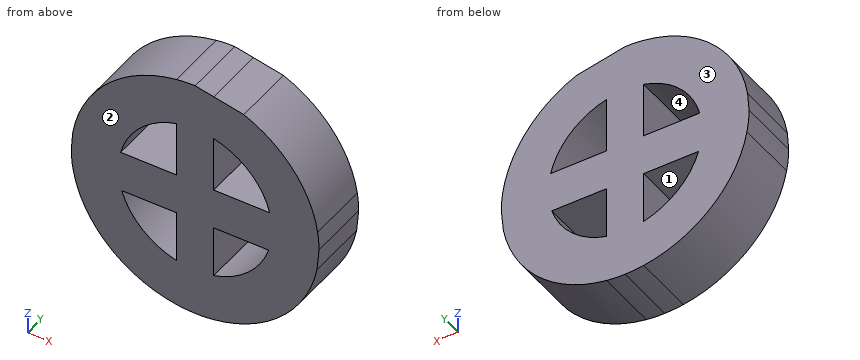
```python
from build123d import *

# Parameters (mm, degrees)
F1_DEPTH = 25


with BuildPart() as f1:
    # F0 (on Front) → F1 (new body)
    with BuildSketch(Plane.XZ):
        with BuildLine():
            Line((-7.5, 30.0790624854), (-7.5, 49.4342998332))
            ThreePointArc((-7.5, 49.4342998332), (-35.3553390593, 35.3553390593), (-49.4342998332, 7.5))
            Line((-49.4342998332, 7.5), (-30.0790624854, 7.5))
            ThreePointArc((-30.0790624854, 7.5), (-21.9203102168, 21.9203102168), (-7.5, 30.0790624854))
        make_face()
        with BuildLine():
            ThreePointArc((49.4342998332, 7.5), (39.5276683909, 30.6196576007), (19.6180084329, 45.9905832223))
            Line((19.6180084329, 45.9905832223), (7.5, 48.4671927359))
            Line((7.5, 48.4671927359), (7.5, 30.0790624854))
            ThreePointArc((7.5, 30.0790624854), (21.9203102168, 21.9203102168), (30.0790624854, 7.5))
            Line((30.0790624854, 7.5), (49.4342998332, 7.5))
        make_face()
        with BuildLine():
            ThreePointArc((7.5, -49.4342998332), (34.773891693, -35.9273775348), (49.1633315746, -9.1086128737))
            Line((49.1633315746, -9.1086128737), (29.631624517, -9.1086128737))
            ThreePointArc((29.631624517, -9.1086128737), (21.322038459, -22.502681528), (7.5, -30.0790624854))
            Line((7.5, -30.0790624854), (7.5, -49.4342998332))
        make_face()
        with BuildLine():
            Line((49.1633315746, -9.1086128737), (50, 0))
            Line((50, 0), (31, 0))
            ThreePointArc((31, 0), (30.6559974559, -4.6054120322), (29.631624517, -9.1086128737))
            Line((29.631624517, -9.1086128737), (49.1633315746, -9.1086128737))
        make_face()
        with BuildLine():
            ThreePointArc((50, 0), (49.8583743801, 3.7606520937), (49.4342998332, 7.5))
            Line((49.4342998332, 7.5), (30.0790624854, 7.5))
            ThreePointArc((30.0790624854, 7.5), (30.7689042464, 3.7781650939), (31, 0))
            Line((31, 0), (50, 0))
        make_face()
        with BuildLine():
            Line((7.5, 48.4671927359), (0, 50))
            Line((0, 50), (0, 31))
            ThreePointArc((0, 31), (3.7781650939, 30.7689042464), (7.5, 30.0790624854))
            Line((7.5, 30.0790624854), (7.5, 48.4671927359))
        make_face()
        with BuildLine():
            Line((-30.0790624854, 7.5), (-49.4342998332, 7.5))
            Line((-49.4342998332, 7.5), (-50, 0))
            Line((-50, 0), (-31, 0))
            ThreePointArc((-31, 0), (-30.7689042464, 3.7781650939), (-30.0790624854, 7.5))
        make_face()
        with BuildLine():
            Line((-31, 0), (-50, 0))
            ThreePointArc((-50, 0), (-49.790393545, -4.5734790515), (-49.1633315746, -9.1086128737))
            Line((-49.1633315746, -9.1086128737), (-29.631624517, -9.1086128737))
            ThreePointArc((-29.631624517, -9.1086128737), (-30.6559974559, -4.6054120322), (-31, 0))
        make_face()
        with BuildLine():
            Line((-29.631624517, -9.1086128737), (-49.1633315746, -9.1086128737))
            ThreePointArc((-49.1633315746, -9.1086128737), (-34.773891693, -35.9273775348), (-7.5, -49.4342998332))
            Line((-7.5, -49.4342998332), (-7.5, -30.0790624854))
            ThreePointArc((-7.5, -30.0790624854), (-21.322038459, -22.502681528), (-29.631624517, -9.1086128737))
        make_face()
        with BuildLine():
            Line((-7.5, -30.0790624854), (-7.5, -49.4342998332))
            ThreePointArc((-7.5, -49.4342998332), (-3.7606520937, -49.8583743801), (0, -50))
            Line((0, -50), (0, -31))
            ThreePointArc((0, -31), (-3.7781650939, -30.7689042464), (-7.5, -30.0790624854))
        make_face()
        with BuildLine():
            ThreePointArc((0, -50), (3.7606520937, -49.8583743801), (7.5, -49.4342998332))
            Line((7.5, -49.4342998332), (7.5, -30.0790624854))
            ThreePointArc((7.5, -30.0790624854), (3.7781650939, -30.7689042464), (0, -31))
            Line((0, -31), (0, -50))
        make_face()
        with BuildLine():
            Line((0, 31), (0, 50))
            ThreePointArc((0, 50), (-3.7606520937, 49.8583743801), (-7.5, 49.4342998332))
            Line((-7.5, 49.4342998332), (-7.5, 30.0790624854))
            ThreePointArc((-7.5, 30.0790624854), (-3.7781650939, 30.7689042464), (0, 31))
        make_face()
        with BuildLine():
            Line((-7.5, 7.5), (-30.0790624854, 7.5))
            ThreePointArc((-30.0790624854, 7.5), (-30.7689042464, 3.7781650939), (-31, 0))
            Line((-31, 0), (-7.5, 0))
            Line((-7.5, 0), (-7.5, 7.5))
        make_face()
        with BuildLine():
            Line((-7.5, -9.1086128737), (-7.5, 0))
            Line((-7.5, 0), (-31, 0))
            ThreePointArc((-31, 0), (-30.6559974559, -4.6054120322), (-29.631624517, -9.1086128737))
            Line((-29.631624517, -9.1086128737), (-7.5, -9.1086128737))
        make_face()
        with BuildLine():
            ThreePointArc((31, 0), (30.7689042464, 3.7781650939), (30.0790624854, 7.5))
            Line((30.0790624854, 7.5), (7.5, 7.5))
            Line((7.5, 7.5), (7.5, 0))
            Line((7.5, 0), (31, 0))
        make_face()
        with BuildLine():
            Line((31, 0), (7.5, 0))
            Line((7.5, 0), (7.5, -9.1086128737))
            Line((7.5, -9.1086128737), (29.631624517, -9.1086128737))
            ThreePointArc((29.631624517, -9.1086128737), (30.6559974559, -4.6054120322), (31, 0))
        make_face()
        with BuildLine():
            ThreePointArc((7.5, 0), (5.3033008589, 5.3033008589), (0, 7.5))
            Line((0, 7.5), (0, 2.5))
            ThreePointArc((0, 2.5), (1.767766953, 1.767766953), (2.5, 0))
            Line((2.5, 0), (7.5, 0))
        make_face()
        with BuildLine():
            Line((0, 2.5), (0, 7.5))
            ThreePointArc((0, 7.5), (-5.3033008589, 5.3033008589), (-7.5, 0))
            Line((-7.5, 0), (-2.5, 0))
            ThreePointArc((-2.5, 0), (-1.767766953, 1.767766953), (0, 2.5))
        make_face()
        with BuildLine():
            ThreePointArc((0, -7.5), (5.3033008589, -5.3033008589), (7.5, 0))
            Line((7.5, 0), (2.5, 0))
            ThreePointArc((2.5, 0), (1.767766953, -1.767766953), (0, -2.5))
            Line((0, -2.5), (0, -7.5))
        make_face()
        with BuildLine():
            Line((-2.5, 0), (-7.5, 0))
            ThreePointArc((-7.5, 0), (-5.3033008589, -5.3033008589), (0, -7.5))
            Line((0, -7.5), (0, -2.5))
            ThreePointArc((0, -2.5), (-1.767766953, -1.767766953), (-2.5, 0))
        make_face()
        with BuildLine():
            Line((0, 0), (-2.5, 0))
            ThreePointArc((-2.5, 0), (-1.767766953, -1.767766953), (0, -2.5))
            Line((0, -2.5), (0, 0))
        make_face()
        with BuildLine():
            ThreePointArc((0, -2.5), (1.767766953, -1.767766953), (2.5, 0))
            Line((2.5, 0), (0, 0))
            Line((0, 0), (0, -2.5))
        make_face()
        with BuildLine():
            ThreePointArc((2.5, 0), (1.767766953, 1.767766953), (0, 2.5))
            Line((0, 2.5), (0, 0))
            Line((0, 0), (2.5, 0))
        make_face()
        with BuildLine():
            Line((0, 0), (0, 2.5))
            ThreePointArc((0, 2.5), (-1.767766953, 1.767766953), (-2.5, 0))
            Line((-2.5, 0), (0, 0))
        make_face()
        with BuildLine():
            Line((7.5, 7.5), (0, 7.5))
            ThreePointArc((0, 7.5), (5.3033008589, 5.3033008589), (7.5, 0))
            Line((7.5, 0), (7.5, 7.5))
        make_face()
        with BuildLine():
            ThreePointArc((-7.5, 0), (-5.3033008589, 5.3033008589), (0, 7.5))
            Line((0, 7.5), (-7.5, 7.5))
            Line((-7.5, 7.5), (-7.5, 0))
        make_face()
        with BuildLine():
            ThreePointArc((0, -7.5), (-5.3033008589, -5.3033008589), (-7.5, 0))
            Line((-7.5, 0), (-7.5, -9.1086128737))
            Line((-7.5, -9.1086128737), (0, -9.1086128737))
            Line((0, -9.1086128737), (0, -7.5))
        make_face()
        with BuildLine():
            Line((7.5, -9.1086128737), (7.5, 0))
            ThreePointArc((7.5, 0), (5.3033008589, -5.3033008589), (0, -7.5))
            Line((0, -7.5), (0, -9.1086128737))
            Line((0, -9.1086128737), (7.5, -9.1086128737))
        make_face()
        with BuildLine():
            Line((0, 7.5), (0, 31))
            ThreePointArc((0, 31), (-3.7781650939, 30.7689042464), (-7.5, 30.0790624854))
            Line((-7.5, 30.0790624854), (-7.5, 7.5))
            Line((-7.5, 7.5), (0, 7.5))
        make_face()
        with BuildLine():
            ThreePointArc((7.5, 30.0790624854), (3.7781650939, 30.7689042464), (0, 31))
            Line((0, 31), (0, 7.5))
            Line((0, 7.5), (7.5, 7.5))
            Line((7.5, 7.5), (7.5, 30.0790624854))
        make_face()
        with BuildLine():
            Line((0, -9.1086128737), (-7.5, -9.1086128737))
            Line((-7.5, -9.1086128737), (-7.5, -30.0790624854))
            ThreePointArc((-7.5, -30.0790624854), (-3.7781650939, -30.7689042464), (0, -31))
            Line((0, -31), (0, -9.1086128737))
        make_face()
        with BuildLine():
            Line((7.5, -30.0790624854), (7.5, -9.1086128737))
            Line((7.5, -9.1086128737), (0, -9.1086128737))
            Line((0, -9.1086128737), (0, -31))
            ThreePointArc((0, -31), (3.7781650939, -30.7689042464), (7.5, -30.0790624854))
        make_face()
    extrude(amount=F1_DEPTH)


solid = f1.part
```
Geometry: final body of the model. Coordinates: model frame, mm. Face numbers are marked on the shaded views. A direction names the side the tool comes from. Give positions to 0.01 mm unless a question says otherwise; leave off trailing zeros. Write each loop counter-clockwise with the first axis right and the second up, starting at its lowest first coordinate (ties: lowest second). Pieces come first, ordered by that corner, then holes.
1. Draft query along Z for the marked faces 3 and 4. Return one class per face: released by +Z, released by -Z, zero draft, split by the parting line, or undercut.
2. Pin query (flat end, axial travel): P1, Ø11, axis at x = -15, y = -7.5, coming from the -Z side; P2, Ø3, axis at y = -14, z = 15.5, coming from the -X side; P3, Ø5, axis at y = -17.5, z = 33, coming from the -X side; P4, Ø5, axis at x = -27.5, z = 13, coming from the -Y side. Return the tip coordinate at first contact, or that it passes through.
3. Section query C-C, the plane z = 18. Return loops of the section in (x, y), then the cut area to 3 significant figures.
4. Section query B-B, the plane x = 23. Return loops of the section in (y, z).
5. Line query: probe 1 along Z at (x, y) = (-24.5, -13.5); probe 2 along Z at (x, y) = (-20, -15); probe 3 along X at (y, z) = (-20.25, 18.5). Output: solid intervals per line, ascending.
6. Section query A-A, the plane y = -1.25. Return loops of the section in (x, z), then the cut area to 3 significant figures.
7. Section query D-D, the plane x = 40. Return loops of the section in (y, z).
8. Reachability of the marked faces 1 and 2 from +Z, -Z, +X, -X, +Y, -Y: full face, straight path, thin tool, end or side. Return the list, or none.
Computed:
1. face 3: zero draft
1. face 4: undercut
2. P1: stops at z = -49.09
2. P2: stops at x = -48
2. P3: stops at x = -39.62
2. P4: stops at y = -25
3. outline: (-46.65, -25) - (-25.24, -25) - (-25.24, 0) - (-46.65, 0) - close; (-7.5, -25) - (7.5, -25) - (7.5, 0) - (-7.5, 0) - close; (25.24, -25) - (46.65, -25) - (46.65, 0) - (25.24, 0) - close
3. area: 1,450 mm2
4. outline: (-25, -44.4) - (0, -44.4) - (0, -20.78) - (-25, -20.78) - close; (-25, -9.11) - (0, -9.11) - (0, 7.5) - (-25, 7.5) - close; (-25, 20.78) - (0, 20.78) - (0, 44.4) - (-25, 44.4) - close
5. probe 1: z = -43.59 to -18.99, -9.11 to 7.5, 18.99 to 43.59
5. probe 2: z = -45.83 to -23.69, -9.11 to 7.5, 23.69 to 45.83
5. probe 3: x = -46.45 to -24.87, -7.5 to 7.5, 24.87 to 46.45
6. outline: (-50, 0) arc R50 ccw to (49.16, -9.11) - (50, 0) arc R50 ccw to (19.62, 45.99) - (0, 50) arc R50 ccw to (-49.43, 7.5) - close; hole (-30.08, 7.5) - (-7.5, 7.5) - (-7.5, 30.08) arc R31 ccw to start; hole (-29.63, -9.11) arc R31 ccw to (-7.5, -30.08) - (-7.5, -9.11) - close; hole (7.5, -30.08) arc R31 ccw to (29.63, -9.11) - (7.5, -9.11) - close; hole (7.5, 7.5) - (30.08, 7.5) arc R31 ccw to (7.5, 30.08) - close
6. area: 6,510 mm2
7. outline: (-25, -30) - (0, -30) - (0, 30) - (-25, 30) - close
8. face 1: +Y, -Y
8. face 2: +Z, -Z, +X, -X, -Y
